Source: CAD feature listing. Evaluate the final solid. Frame: model axes, mm. Face numbers are marked on the shaded views. A direction names the side the tool comes from. Give positions to 0.01 mm unless a question says otherwise; leave off trailing zeros. Loops run counter-clockwise (first coordinate to the right, second up) from the corner with the lowest first, then second, coordinate; pieces in that order, holes last. Notation, with made-up numbers: M 41,-34.5 L 71,-34.5 A18 ccw 71,-12.5 Z; hole C 0,-38 d10. An arc over 180 degrees is marked long. Write item = value, one per line.
from build123d import *

# Parameters (mm, degrees)
SKETCH1_R      = 3.175
EXTRUDE1_DEPTH = 1.8542
FILLET1_R      = 1.524
SKETCH2_R      = 1.7526
EXTRUDE2_DEPTH = 9.525
EXTRUDE3_DEPTH = 1.016


with BuildPart() as part:
    # Sketch1 → Extrude1 (new body)
    with BuildSketch(Plane.XY):
        Circle(SKETCH1_R)
    extrude(amount=EXTRUDE1_DEPTH)

    # Fillet1
    fillet1_edges = [part.edges().sort_by_distance(p)[0] for p in [
        (-3.175, 0, 0),
    ]]
    fillet(fillet1_edges, radius=FILLET1_R)

    # Sketch2 → Extrude2 (add)
    with BuildSketch(Plane.XY.offset(1.8542)):
        Circle(SKETCH2_R)
    extrude(amount=EXTRUDE2_DEPTH)

    # Sketch3 → Extrude3 (cut)
    with BuildSketch(Plane(origin=(0, 0, 0), x_dir=(-1, 0, 0), z_dir=(0, 0, -1))):
        Polygon((0.59085384, 0.981566666), (-0.554634748, 1.002477769), (-1.145488588, 0.020911103), (-0.59085384, -0.981566666), (0.554634748, -1.002477769), (1.145488588, -0.020911103), align=None)
    extrude(amount=-EXTRUDE3_DEPTH, mode=Mode.SUBTRACT)


solid = part.part
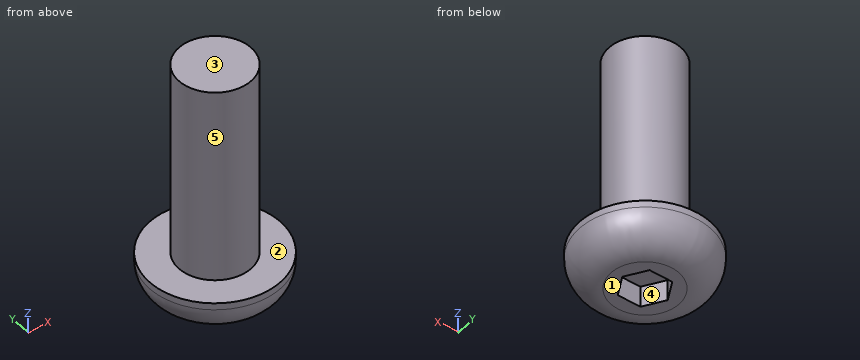
1. Cut plane A-A, the plane x = 0. Return the cut outline in (y, z) (3 decimals).
Derived:
outline = M -3.175,1.524 A1.524 ccw -1.651,0 L -0.992,0 L -0.992,1.016 L 0.992,1.016 L 0.992,0 L 1.651,0 A1.524 ccw 3.175,1.524 L 3.175,1.854 L 1.753,1.854 L 1.753,11.379 L -1.753,11.379 L -1.753,1.854 L -3.175,1.854 Z
2. First-contact query: pin 1 Ø1 at (y, z) = (-0.5, 10) entering from +X; pin 2 Ø1 at (x, z) = (1, 6) entering from +Y; pin 3 Ø1 at (x, y) = (-0.5, 0.5) entering from -Z; pin 4 Ø3 at (x, z) = (-0.5, 3.5) entering from +Y. Flat tips, straight axial feed; report the tip coordinate or a pass-through.
Derived:
pin_1 = 1.75
pin_2 = 1.68
pin_3 = 0
pin_4 = 1.75
3. Cut plane B-B, the plane z = 9.5. Return the cut outline in (x, y), then the cut area to 3 significant figures.
Derived:
outline = C 0,0 d3.51
area = 9.65 mm²
4. Material intervals for probe 1 along Z at (x, y) = (0.5, 2); probe 2 along Y at (x, z) = (1.25, 6); probe 3 along Y at (x, z) = (0.5, 9), sorted ascending. Write a range as from..to.
Derived:
probe_1 = 0.06..1.85
probe_2 = -1.23..1.23
probe_3 = -1.68..1.68
5. Reachability of the marked faces 1 and 2 from +Z, -Z, +X, -X, +Y, -Y: full face, straight path, thin tool, end or side. Return the list, or none.
Derived:
face_1 = -Z, +X, -X, +Y, -Y
face_2 = +Z
6. Pull-direction query (Y, two-part tool) for the marked faces 3, 4 and 5; classes: +Y half, -Y half, draft (parallel to the pull), parting line (faces both ways), or undercut.
Derived:
face_3 = draft
face_4 = undercut
face_5 = parting line
